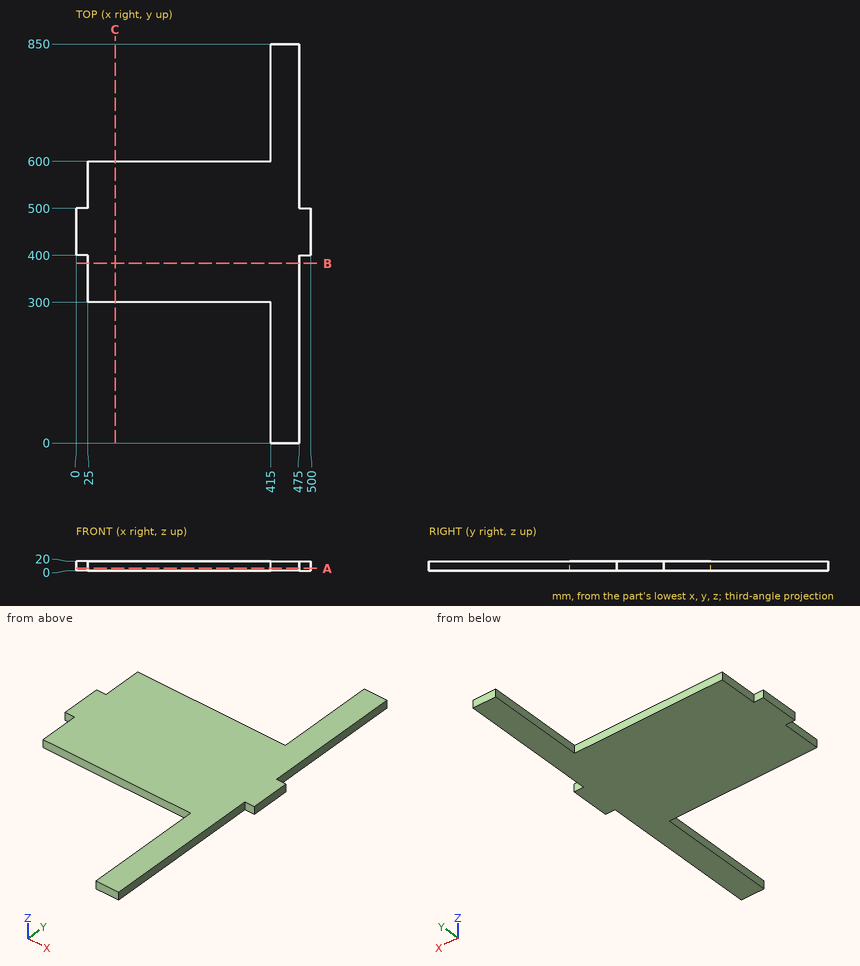
Verification items for this drawing (mm, ordinates from the low corner). Give positions to 0.01 mm unless a question says otherwise; leave off trailing zeros. Loops run counter-clockwise (first coordinate to the right, second up) from the corner with the lowest first, then second, coordinate; pieces in that order, holes last. Notation, with made-up numbers: M 73.25,3 L 126.25,3 A24 ccw 126.25,13 Z; hole C 31,48 d6. An arc over 180 degrees is marked long. Answer as CSV lines item,"result".
Item 1: Depth check by flat-ended pin: P1, Ø6, axis at x = 6.5, z = 7, coming from the +Y side; P2, Ø10, axis at y = 182, z = 7, coming from the -X side; P3, Ø10, axis at y = 367, z = 13, coming from the -X side. Enter the tip coordinate at first touch or a pass-through.
Values:
P1,"stops at y = 500"
P2,"stops at x = 415"
P3,"stops at x = 25"
Item 2: Cross-section at C-C on x = 83.5. Record the cut outline in (y, z).
Values:
outline,"M 300,0 L 600,0 L 600,20 L 300,20 Z"
Item 3: Cross-section at B-B on y = 383. Record the cut outline in (x, z).
Values:
outline,"M 25,0 L 475,0 L 475,20 L 25,20 Z"
Item 4: Cross-section at A-A on z = 4.75. Record the cut outline in (x, y).
Values:
outline,"M 0,400 L 25,400 L 25,300 L 415,300 L 415,0 L 475,0 L 475,400 L 500,400 L 500,500 L 475,500 L 475,850 L 415,850 L 415,600 L 25,600 L 25,500 L 0,500 Z"
Item 5: Material ranges on line 1 (X direction, y = 175, z = 4); line 2 (Y direction, x = 251.5, z = 10); line 3 (X direction, y = 350, z = 10.5), recorded low to high.
Values:
line 1,"x = 415 to 475"
line 2,"y = 300 to 600"
line 3,"x = 25 to 475"
